Geometry check sheet. Reference: the model listing, model coordinates, mm. A direction names the side the tool comes from. Give positions to 0.01 mm unless a question says otherwise; leave off trailing zeros. Loops run counter-clockwise (first coordinate to the right, second up) from the corner with the lowest first, then second, coordinate; pieces in that order, holes last. Notation, with made-up numbers: (64.5, 47.25) -> (103.5, 47.25) arc R16 ccw to (103.5, 61.25) -> close; hole circle Ø11 at (11.25, 26.5). An arc over 180 degrees is marked (long way). One line per question, with ' | ' between items.
from build123d import *

# Parameters (mm, degrees)
F1_DEPTH = 6.096
F4_R     = 2.54
F5_R     = 1.27
F6_W     = 9.525
F6_H     = 5.969
F7_DEPTH = 6.097


# Not quite as in the source:
# - a feature of the source that left no trace in its solid (it failed there, or was rolled back) is left out


with BuildPart() as f1:
    # F0 (on Front) → F1 (new body)
    with BuildSketch(Plane.XZ):
        Polygon((-6.35, 0), (0, 0), (0, 12.7), (12.2428, 12.7), (12.2428, -3.175), (313.8678, -3.175), (313.8678, 12.7), (319.8368, 12.7), (319.8368, 7.62), (345.2368, 19.05), (43.434, 58.42), (0, 22.225), (-11.43, 12.7), align=None)
    extrude(amount=F1_DEPTH)

    # F4
    f4_edges = [f1.edges().sort_by_distance(p)[0] for p in [
        (43.434, -3.048, 58.42),
        (-11.43, -3.048, 12.7),
        (-6.35, -3.048, 0),
        (345.2368, -3.048, 19.05),
    ]]
    fillet(f4_edges, radius=F4_R)

    # F5
    f5_edges = [f1.edges().sort_by_distance(p)[0] for p in [
        (0, -3.048, 0),
        (12.2428, -3.048, -3.175),
        (319.8368, -3.048, 7.62),
        (313.8678, -3.048, -3.175),
    ]]
    fillet(f5_edges, radius=F5_R)

    # F6 (on face) → F7 (cut, through all)
    with BuildSketch(Plane.XZ.offset(6.096)):
        with Locations((23.3553, 6.1595)):
            Rectangle(F6_W, F6_H)
        with Locations((302.7553, 6.1595)):
            Rectangle(F6_W, F6_H)
    extrude(amount=-F7_DEPTH, mode=Mode.SUBTRACT)


solid = f1.part
Item 1: Set-up check for faces 1 (the face through (12.243, -3, 5)), 2 (the face through (303, -3, 3.175)), 3 (the face through (329.24, -3.01, 11.85)): record each of +Z, -Z, +X, -X, +Y, -Y from which the full face is reachable in a straight line by a thin tool's end or side.
Result:
face 1: -Z, +Y, -Y | face 2: +Y, -Y | face 3: -Z, +X, +Y, -Y
Item 2: Sectioned sample at A-A (y = -4.5). Record the cut outline in (x, z) (3 decimals).
Result:
outline: (-10.745, 10.987) -> (-6.989, 1.597) arc R2.54 ccw to (-4.63, 0) -> (-1.27, 0) arc R1.27 ccw to (0, 1.27) -> (0, 12.7) -> (12.243, 12.7) -> (12.243, -1.905) arc R1.27 ccw to (13.513, -3.175) -> (312.598, -3.175) arc R1.27 ccw to (313.868, -1.905) -> (313.868, 12.7) -> (319.837, 12.7) -> (319.837, 9.584) arc R1.27 ccw to (321.628, 8.426) -> (337.068, 15.374) arc R2.54 ccw to (336.354, 20.209) -> (44.535, 58.276) arc R2.54 ccw to (42.581, 57.709) -> (-10.012, 13.881) arc R2.54 ccw to start; hole (18.593, 3.175) -> (28.118, 3.175) -> (28.118, 9.144) -> (18.593, 9.144) -> close; hole (297.993, 3.175) -> (307.518, 3.175) -> (307.518, 9.144) -> (297.993, 9.144) -> close
Item 3: Sectioned sample at C-C (z = 49.5). Record the cut outline in (x, y), plus the area to 3 significant figures.
Result:
outline: (32.73, -6.1) -> (111.81, -6.1) -> (111.81, 0) -> (32.73, 0) -> close | area: 482 mm2
Item 4: Sectioned sample at B-B (x = 113.5). Record the cut outline in (y, z) (3 decimals), plus the area to 3 significant figures.
Result:
outline: (-6.096, -3.175) -> (0, -3.175) -> (0, 49.28) -> (-6.096, 49.28) -> close | area: 320 mm2
Item 5: Depth check by flat-ended pin: pin 1 Ø1.6 at (y, z) = (-3, 11) entering from -X; pin 2 Ø3 at (x, y) = (304, -1.5) entering from +Z (3 decimals); pin 3 Ø2.5 at (x, y) = (-3.5, -4.5) entering from -Z. Enter the tip coordinate at first touch or a pass-through.
Result:
pin 1: x = -10.92 | pin 2: z = 24.625 | pin 3: z = 0
Item 6: Scan lines: probe 1 along X at (y, z) = (-5.5, 12.5); probe 2 along Z at (x, y) = (307, -0.5) (3 decimals); probe 3 along Z at (x, y) = (19.5, -2.25) (3 decimals). Record each from-to range of solid material in increasing order.
Result:
probe 1: -10.86 to 0, 12.24 to 313.87, 319.84 to 330.68 | probe 2: -3.175 to 3.175, 9.144 to 24.038 | probe 3: -3.175 to 3.175, 9.144 to 38.475
Item 7: Release check for a two-part mould opening along X. For faces 4 (the face through (297.993, -3, 6)), 5 (the face through (16.65, -3.01, 36.1)), 6 (the face through (192.487, -3.005, 38.976)) record: pulls with the +X half, pulls with the -X half, needs draft (parallel to the pull), parting line crosses it, or undercut.
Result:
face 4: undercut | face 5: pulls with the -X half | face 6: pulls with the +X half
